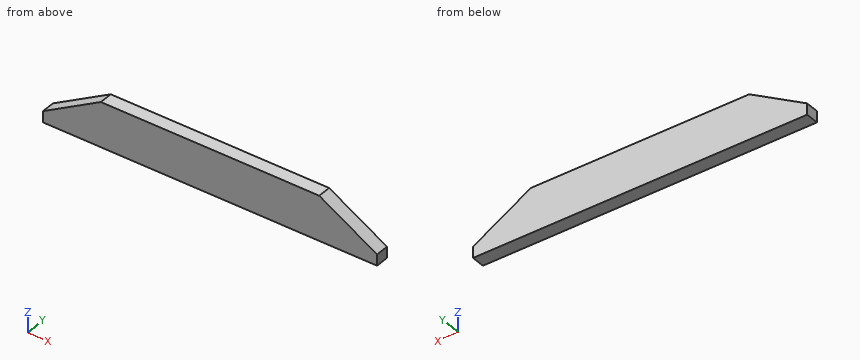
from build123d import *
from OCP.BRepFilletAPI import BRepFilletAPI_MakeChamfer

# Parameters (mm, degrees)
SKETCH_1_W      = 150
SKETCH_1_H      = 6
EXTRUDE_1_DEPTH = 20
CHAMFER_1_SIZE  = 15
CHAMFER_1_SIZE2 = 25.980762114


with BuildPart() as part:
    # Эскиз1 → Бобышка-Вытянуть1 (new body)
    with BuildSketch(Plane.XY):
        with Locations((0, 3)):
            Rectangle(SKETCH_1_W, SKETCH_1_H)
    extrude(amount=EXTRUDE_1_DEPTH)

    # Фаска1: one chamfer whose edges measure the first distance from different faces: ONE call of the kernel's chamfer builder (chamfer() names one face for all edges)
    chamfer_1_edges_1 = [part.edges().sort_by_distance(p)[0] for p in [
        (75, 3, 20),
    ]]
    chamfer_1_side_1 = [part.faces().sort_by_distance(p)[0] for p in [
        (75, 3, 10),
    ]]
    chamfer_1_edges_2 = [part.edges().sort_by_distance(p)[0] for p in [
        (-75, 3, 20),
    ]]
    chamfer_1_side_2 = [part.faces().sort_by_distance(p)[0] for p in [
        (-75, 3, 10),
    ]]
    chamfer_1 = BRepFilletAPI_MakeChamfer(part.part.solid().wrapped)
    for e in chamfer_1_edges_1:
        chamfer_1.Add(CHAMFER_1_SIZE, CHAMFER_1_SIZE2, e.wrapped, chamfer_1_side_1[0].wrapped)  # the first distance lies on this face
    for e in chamfer_1_edges_2:
        chamfer_1.Add(CHAMFER_1_SIZE, CHAMFER_1_SIZE2, e.wrapped, chamfer_1_side_2[0].wrapped)  # the first distance lies on this face
    add(Compound.cast(chamfer_1.Shape()), mode=Mode.REPLACE)


solid = part.part
Read the model definition and answer for the solid it produces. Units are mm, in the model's axes. Coordinates: 2 decimals unless noted, no trailing zeros. Write each loop counter-clockwise with the first axis right and the second up, starting at its lowest first coordinate (ties: lowest second). Pieces come first, ordered by that corner, then holes. Notation, with made-up numbers: (35, -33.75) -> (91, -33.75) arc R31 cw to (91, -7.75) -> close; hole circle Ø2 at (-8, 38). An arc over 180 degrees is marked (long way). Return JSON: item names as keys, results as strings.
(1) Consider line 1 along X through (y, z) = (5.3, 15.5); line 2 along X through (y, z) = (4.9, 16.25); line 3 along Z through (x, y) = (-67.5, 4). Determine where each line is inside the solid, lowest interval first. Write a range as from..to.
Answers below:
{"line 1": "-56.81..56.81", "line 2": "-55.51..55.51", "line 3": "0..9.33"}
(2) The part is cut by section C-C on z = 9. Give the vertices of the cut face in (x, y).
Answers below:
{"outline": "(-68.07, 0) -> (68.07, 0) -> (68.07, 6) -> (-68.07, 6) -> close"}
(3) The part is cut by section A-A on y = 2.9. Give the vertices of the cut face in (x, z), then the cut area to 3 significant figures.
Answers below:
{"outline": "(-75, 0) -> (75, 0) -> (75, 5) -> (49.02, 20) -> (-49.02, 20) -> (-75, 5) -> close", "area": "2,610 mm^2"}
(4) The part is cut by section B-B on z = 14.5. Give the vertices of the cut face in (x, y).
Answers below:
{"outline": "(-58.55, 0) -> (58.55, 0) -> (58.55, 6) -> (-58.55, 6) -> close"}
